Autodesk Inventor part; units mm, degrees
ref_plane "Work Plane1" through (5, 0, 0) normal (1, 0, 0) x (0, 1, 0)
ref_plane "XZ Plane" through (0, 0, 0) normal (0, 1, 0) x (-1, 0, 0)
ref_plane "XY Plane" through (0, 0, 0) normal (0, 0, 1) x (1, 0, 0)
sketch "Sketch1" plane through (0, 0, 0) normal (0, 1, 0) x (-1, 0, 0)
  circle A0 centre (0, 0) radius 6
  dimension "d0" = 12
extrude "Extrusion1" add sketch "Sketch1" along normal blind 2
sketch "Sketch2" plane through (0, 2, 0) normal (0, 1, 0) x (1, 0, 0)
  circle A0 centre (0, 0) radius 4
  circle A1 centre (0, 0) radius 6
  dimension "d3" = 8
extrude "Extrusion2" add sketch "Sketch2" along normal blind 20
sketch "Sketch3" plane through (0, 22, 0) normal (0, 1, 0) x (1, 0, 0)
  arc A0 (-6, 0) -> (0, -6) centre (0, 0) ccw
  circle A1 centre (0, 0) radius 6 construction
  arc A2 (6, 0) -> (0, 6) centre (0, 0) ccw
  line L0 (0, -6) -> (0, -4)
  circle A3 centre (0, 0) radius 4 construction
  line L1 (0, 4) -> (0, 6)
  line L2 (6, 0) -> (4, 0)
  line L3 (-4, 0) -> (-6, 0)
  arc A4 (-4, 0) -> (0, -4) centre (0, 0) ccw
  arc A5 (4, 0) -> (0, 4) centre (0, 0) ccw
extrude "Extrusion3" add sketch "Sketch3" along normal blind 5
ref_plane "Work Plane1" through (5, 0, 0) normal (1, 0, 0) x (0, 1, 0)
sketch "Sketch5" plane through (5, 0, 0) normal (1, 0, 0) x (0, 1, 0)
  line L0 (22, 0) -> (22, 6) construction
  line L1 (22, 6) -> (2, -6) construction
  line L2 (22, -6) -> (22, 0) construction
  line L3 (22, -6) -> (2, 6) construction
  circle A0 centre (12, 0) radius 1.75
  point P0 (0, 0)
  dimension "d10" = 3.5
extrude "Extrusion4" add sketch "Sketch5" along normal blind 12
pattern_circular "Circular Pattern1" count 3 over 360 about axis through (0, 0, 0) along (0, 1, 0) of "Extrusion4"
thread "Thread1"
thread "Thread2"
thread "Thread3"
properties part number "UntererRührerHalter"
Source: CAD feature listing. Evaluate the final solid. Frame: model axes, mm. A direction names the side the tool comes from. Coordinates: 2 decimals unless noted, no trailing zeros. Loops run counter-clockwise (first coordinate to the right, second up) from the corner with the lowest first, then second, coordinate; pieces in that order, holes last. Notation, with made-up numbers: (-27, 54.5) -> (26, 54.5) arc R26 cw to (26, 82.5) -> close; hole circle Ø11 at (32.25, -28). An arc over 180 degrees is marked (long way). Answer in a Markdown table with one row per item. Add a question column.
Q1. Section B-B on y = 12. Return the cut outline in (x, z).
Q2. Ray query, line 1 along X through (y, z) = (15.25, 0); line 2 along Z through (x, y) = (0.25, 2.5); line 3 along Y through (x, z) = (2.5, 3). Return the intervals inside material, ascending.
Q3. Reachability of faces 1 (the face through (5, 24, 0)), 2 (the face through (0, 2, 0)), 3 (the face through (0, 24, -5)), 4 (the face through (-3, 27, 3)), 5 (the face through (11.291, 13.669, -0.526)) from +Z, -Z, +X, -X, +Y, -Y: full face, straight path, thin tool, end or side. Return the list, or none.
Q4. Section A-A on y = 23.75. Return the cut outline in (x, z), and give its area (3 significant figures).
Q5. Pull-direction query (Z, two-part tool) for faces 6 (the face through (-5.19, 13.67, 10.04)), 7 (the face through (-5, 24, 0)), 8 (the face through (0, 24, 5)); classes: pulls with the +Z half, pulls with the -Z half, needs draft (parallel to the pull), parting line crosses it, or undercut.
Q6. Section C-C on z = -0.5. Return the cut outline in (x, y), and give its area (3 significant figures).
Q7. Contact query for flat-ended pins moving along their axis: pin 1 Ø1.6 at (x, y) = (-5.5, 25.5) entering from -Z; pin 2 Ø0.6 at (y, z) = (25.5, -5) entering from -X; pin 3 Ø8 at (x, z) = (12, -1.5) entering from -Y; pin 4 Ø5 at (x, z) = (-3.5, -2) entering from +Y. Output: stop coordinate, or through.
Q8. Section D-D on x = 8.75. Return the cut outline in (y, z), and give its area (3 significant figures).
Computed values:
| question | item | result |
|---|---|---|
| 1 | outline | (-10.02, -13.85) -> (-6.98, -15.6) -> (-1.35, -5.85) arc R6 ccw to (5.74, -1.75) -> (17, -1.75) -> (17, 1.75) -> (5.74, 1.75) arc R6 ccw to (-1.35, 5.85) -> (-6.98, 15.6) -> (-10.02, 13.85) -> (-4.39, 4.1) arc R6 ccw to (-4.39, -4.1) -> close; hole circle Ø8 at (0, 0) |
| 2 | line 1 | x = -6 to -4, 4 to 6 |
| 2 | line 2 | z = -5.99 to -3.99, 3.99 to 5.99 |
| 2 | line 3 | y = 0 to 2 |
| 3 | face 1 | +Z, +X, +Y |
| 3 | face 2 | +Y |
| 3 | face 3 | -Z, -X, +Y |
| 3 | face 4 | +Z, -Z, +X, -X, +Y |
| 3 | face 5 | +X |
| 4 | outline | (-6, 0) -> (-4, 0) arc R4 cw to (0, 4) -> (0, 6) arc R6 ccw to start; (0, -6) arc R6 ccw to (6, 0) -> (4, 0) arc R4 cw to (0, -4) -> close |
| 4 | area | 31.4 mm^2 |
| 5 | face 6 | undercut |
| 5 | face 7 | pulls with the -Z half |
| 5 | face 8 | needs draft |
| 6 | outline | (-5.98, 0) -> (5.98, 0) -> (5.98, 10.32) -> (17, 10.32) -> (17, 13.68) -> (5.98, 13.68) -> (5.98, 27) -> (3.97, 27) -> (3.97, 2) -> (-3.97, 2) -> (-3.97, 22) -> (-5.98, 22) -> close |
| 6 | area | 151 mm^2 |
| 7 | pin 1 | stops at z = 0 |
| 7 | pin 2 | stops at x = 0 |
| 7 | pin 3 | stops at y = 10.25 |
| 7 | pin 4 | stops at y = 27 |
| 8 | outline | circle Ø3.5 at (12, 0) |
| 8 | area | 9.62 mm^2 |
